```python
from build123d import *

# Parameters (mm, degrees)
SKETCH1_R           = 1.5
BOSS_EXTRUDE5_DEPTH = 2.75
BOSS_EXTRUDE6_DEPTH = 16.25
CUT_EXTRUDE2_DEPTH  = 16.25


with BuildPart() as part:
    # Sketch1 → Boss-Extrude5 (new, symmetric)
    # profile 1 of 13: a face of its own
    with BuildSketch(Plane(origin=(0, 0, 0), x_dir=(1, 0, 0), z_dir=(0, 1, 0))):
        Polygon((-15.475330795, -15.475330795), (-4.035534165, -20.213849709), (-20.251928631, -3.943603517), align=None)
    # profile 2 of 13: a face of its own
    with BuildSketch(Plane(origin=(0, 0, 0), x_dir=(1, 0, 0), z_dir=(0, 1, 0))):
        Polygon((20.175206492, -4.128827144), (4.037646201, -20.212974875), (15.475330795, -15.475330795), align=None)
    # profile 3 of 13: a face of its own
    with BuildSketch(Plane(origin=(0, 0, 0), x_dir=(1, 0, 0), z_dir=(0, 1, 0))):
        Polygon((3.904649762, 20.268063804), (20.306578392, 3.811667321), (15.475330795, 15.475330795), align=None)
    # profile 4 of 13: a face of its own
    with BuildSketch(Plane(origin=(0, 0, 0), x_dir=(1, 0, 0), z_dir=(0, 1, 0))):
        Polygon((3.586127609, -20.4), (4.037646201, -20.212974875), (20.175206492, -4.128827144), (20.361356783, -3.679420587), (20.361356783, 3.679420587), (20.306578392, 3.811667321), (3.904649762, 20.268063804), (-3.795350238, 20.268063804), (-20.306707021, 3.811356783), (-20.306707021, -3.811356783), (-20.251928631, -3.943603517), (-4.035534165, -20.213849709), (-3.586127609, -20.4), align=None)
        with Locations(Location((0, 0, 0), (0, 0, 270))):
            Circle(SKETCH1_R, mode=Mode.SUBTRACT)
    # profile 5 of 13: a face of its own
    with BuildSketch(Plane(origin=(0, 0, 0), x_dir=(1, 0, 0), z_dir=(0, 1, 0))):
        Polygon((-15.475330795, 15.475330795), (-20.306707021, 3.811356783), (-3.795350238, 20.268063804), (-3.795350238, 20.313337149), align=None)
    # profile 6 of 13: a face of its own
    with BuildSketch(Plane(origin=(0, 0, 0), x_dir=(1, 0, 0), z_dir=(0, 1, 0))):
        Polygon((-21.885422692, 0), (-20.306707021, -3.811356783), (-20.306707021, 3.811356783), align=None)
    # profile 7 of 13: a face of its own
    with BuildSketch(Plane(origin=(0, 0, 0), x_dir=(1, 0, 0), z_dir=(0, 1, 0))):
        Polygon((-20.306707021, -3.888643217), (-20.306707021, -3.811356783), (-21.885422692, 0), (-20.306707021, 3.811356783), (-34.056707021, 3.811356783), (-34.056707021, -3.888643217), align=None)
    # profile 8 of 13: a face of its own
    with BuildSketch(Plane(origin=(0, 0, 0), x_dir=(1, 0, 0), z_dir=(0, 1, 0))):
        Polygon((3.85, -34.15), (3.85, -20.4), (3.586127609, -20.4), (0, -21.885422692), (-3.586127609, -20.4), (-3.85, -20.4), (-3.85, -34.15), align=None)
    # profile 9 of 13: a face of its own
    with BuildSketch(Plane(origin=(0, 0, 0), x_dir=(1, 0, 0), z_dir=(0, 1, 0))):
        Polygon((0, -21.885422692), (3.586127609, -20.4), (-3.586127609, -20.4), align=None)
    # profile 10 of 13: a face of its own
    with BuildSketch(Plane(origin=(0, 0, 0), x_dir=(1, 0, 0), z_dir=(0, 1, 0))):
        Polygon((20.361356783, 3.679420587), (20.361356783, -3.679420587), (21.885422692, 0), align=None)
    # profile 11 of 13: a face of its own
    with BuildSketch(Plane(origin=(0, 0, 0), x_dir=(1, 0, 0), z_dir=(0, 1, 0))):
        Polygon((-3.795350238, 20.268063804), (3.904649762, 20.268063804), (0, 21.885422692), (-3.795350238, 20.313337149), align=None)
    # profile 12 of 13: a face of its own
    with BuildSketch(Plane(origin=(0, 0, 0), x_dir=(1, 0, 0), z_dir=(0, 1, 0))):
        Polygon((0, 21.885422692), (3.904649762, 20.268063804), (3.904649762, 34.018063804), (-3.795350238, 34.018063804), (-3.795350238, 20.313337149), align=None)
    # profile 13 of 13: a face of its own
    with BuildSketch(Plane(origin=(0, 0, 0), x_dir=(1, 0, 0), z_dir=(0, 1, 0))):
        Polygon((20.361356783, -3.679420587), (20.361356783, -3.943292979), (34.111356783, -3.943292979), (34.111356783, 3.756707021), (20.361356783, 3.756707021), (20.361356783, 3.679420587), (21.885422692, 0), align=None)
    extrude(amount=BOSS_EXTRUDE5_DEPTH, both=True)

    # Sketch1_10 → Boss-Extrude6 (add)
    with BuildSketch(Plane(origin=(0, 0, 0), x_dir=(1, 0, 0), z_dir=(0, 1, 0))):
        Polygon((0, -21.885422692), (3.586127609, -20.4), (-3.586127609, -20.4), align=None)
        Polygon((3.85, -34.15), (3.85, -20.4), (3.586127609, -20.4), (0, -21.885422692), (-3.586127609, -20.4), (-3.85, -20.4), (-3.85, -34.15), align=None)
        Polygon((-20.306707021, -3.888643217), (-20.306707021, -3.811356783), (-21.885422692, 0), (-20.306707021, 3.811356783), (-34.056707021, 3.811356783), (-34.056707021, -3.888643217), align=None)
        Polygon((-21.885422692, 0), (-20.306707021, -3.811356783), (-20.306707021, 3.811356783), align=None)
        Polygon((-3.795350238, 20.268063804), (3.904649762, 20.268063804), (0, 21.885422692), (-3.795350238, 20.313337149), align=None)
        Polygon((0, 21.885422692), (3.904649762, 20.268063804), (3.904649762, 34.018063804), (-3.795350238, 34.018063804), (-3.795350238, 20.313337149), align=None)
        Polygon((20.361356783, 3.679420587), (20.361356783, -3.679420587), (21.885422692, 0), align=None)
        Polygon((20.361356783, -3.679420587), (20.361356783, -3.943292979), (34.111356783, -3.943292979), (34.111356783, 3.756707021), (20.361356783, 3.756707021), (20.361356783, 3.679420587), (21.885422692, 0), align=None)
    extrude(amount=BOSS_EXTRUDE6_DEPTH)

    # Sketch3 → Cut-Extrude2 (cut)
    with BuildSketch(Plane(origin=(0, 0, -3.756707021), x_dir=(-1, 0, 0), z_dir=(0, 0, -1))):
        Polygon((-30.361356783, -2.75), (-34.111356783, 16.25), (-34.111356783, -2.75), align=None)
    extrude(amount=-CUT_EXTRUDE2_DEPTH, mode=Mode.SUBTRACT)


solid = part.part
```
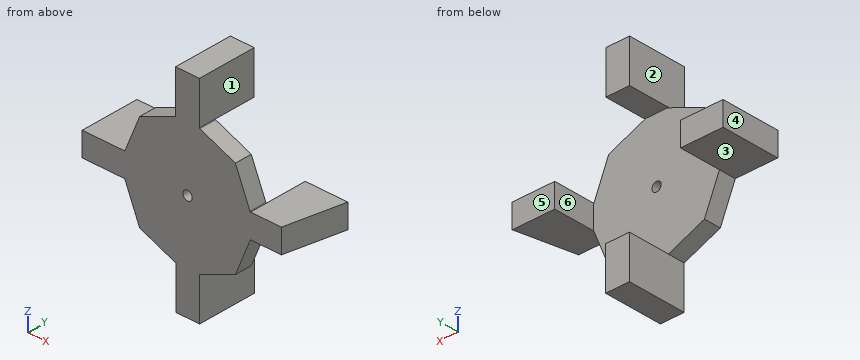
Here's how the part is built. I have some questions about the finished solid (model axes, mm). Face numbers are marked on the shaded views. A direction names the side the tool comes from. Round coordinates to 2 decimals unless told otherwise and drop trailing zeros. Order: outer loops, then holes, each group sorted by start corner. A loop starts at its lowest first (then second) coordinate and runs counter-clockwise, first axis right, second up. Notation, with made-up numbers: M 53,-5 L 72,-5 A16 ccw 72,15 Z; hole C 2.5,25 d10. An arc over 180 degrees is marked long. Answer in a Markdown table with one row per item.
Item 1: I'm going to push flat-ended pins straight in: pin 1 (4 mm diameter, centred on y = 5.5, z = -25, fed in from +X); pin 2 (4 mm diameter, centred on y = 1.5, z = -9, fed in from +X); pin 3 (1 mm diameter, centred on x = 9, z = 17, fed in from +Y). Where does each tip first touch, or does it pass through?
A:
| item | result |
|---|---|
| pin 1 | stops at x = 3.9 |
| pin 2 | stops at x = 18.99 |
| pin 3 | stops at y = 2.75 |
Item 2: For the marked faces 1, 2 and 3, which set-ups out of +Z, -Z, +X, -X, +Y, -Y let a thin tool reach every point of the face, with its end or its side?
A:
| item | result |
|---|---|
| face 1 | +Z, +X, +Y, -Y |
| face 2 | +Z, -X, +Y, -Y |
| face 3 | -Z, -X, +Y, -Y |
Item 3: Imagine slicing it at A-A, the plane x = 0. Write out the boundary of the cut face in (y, z).
A:
| item | result |
|---|---|
| outline | M -2.75,-34.02 L 16.25,-34.02 L 16.25,-20.27 L 2.75,-20.27 L 2.75,-1.5 L -2.75,-1.5 Z; M -2.75,1.5 L 2.75,1.5 L 2.75,20.4 L 16.25,20.4 L 16.25,34.15 L -2.75,34.15 Z |
Item 4: Imagine slicing it at D-D, the plane y = -1.25. Write out the boundary of the cut face in (x, z), and give its area (3 significant figures).
A:
| item | result |
|---|---|
| outline | M -34.06,-3.81 L -20.31,-3.81 L -15.48,-15.48 L -3.8,-20.31 L -3.8,-34.02 L 3.9,-34.02 L 3.9,-20.27 L 15.48,-15.48 L 20.36,-3.68 L 20.36,-3.76 L 30.66,-3.76 L 30.66,3.94 L 20.36,3.94 L 20.36,3.68 L 15.48,15.48 L 3.59,20.4 L 3.85,20.4 L 3.85,34.15 L -3.85,34.15 L -3.85,20.4 L -3.59,20.4 L -15.48,15.48 L -20.31,3.81 L -20.31,3.89 L -34.06,3.89 Z; hole C 0,0 d3 |
| area | 1,720 mm2 |
Item 5: Thinking about a two-plate mould opening in X: for the marked faces 4, 5 and 6, which applies, +X half, -X half, draft (parallel to the pull), parting line (faces both ways), or undercut?
A:
| item | result |
|---|---|
| face 4 | -X half |
| face 5 | draft |
| face 6 | undercut |
Item 6: Imagine slicing it at B-B, the plane z = 0. Write out the boundary of the cut face in (x, y), and give its area (3 significant figures).
A:
| item | result |
|---|---|
| outline | M -34.06,-2.75 L -1.5,-2.75 L -1.5,2.75 L -20.31,2.75 L -20.31,16.25 L -34.06,16.25 Z; M 1.5,-2.75 L 30.36,-2.75 L 34.11,16.25 L 20.36,16.25 L 20.36,2.75 L 1.5,2.75 Z |
| area | 694 mm2 |
Item 7: Imagine slicing it at C-C, the plane y = 7.5. Write out the boundary of the cut face in (x, z).
A:
| item | result |
|---|---|
| outline | M -34.06,-3.81 L -20.31,-3.81 L -20.31,3.89 L -34.06,3.89 Z; M -3.85,20.4 L 3.85,20.4 L 3.85,34.15 L -3.85,34.15 Z; M -3.8,-34.02 L 3.9,-34.02 L 3.9,-20.27 L -3.8,-20.27 Z; M 20.36,-3.76 L 32.38,-3.76 L 32.38,3.94 L 20.36,3.94 Z |
Item 8: If I drill on L1, parallel to Z at x = -30, y = 8.75; L2, parallel to X at y = 2.5, z = 23.5; L3, parallel to Y at x = -17, z = 8, over which ranges is the centre line in solid material (lowest first)? Write a range as from..to.
A:
| item | result |
|---|---|
| L1 | z = -3.81..3.89 |
| L2 | x = -3.85..3.85 |
| L3 | y = -2.75..2.75 |
